Here's how the part is built. I have some questions about the finished solid (model axes, mm). A direction names the side the tool comes from. Coordinates: 2 decimals unless noted, no trailing zeros. Write each loop counter-clockwise with the first axis right and the second up, starting at its lowest first coordinate (ties: lowest second). Pieces come first, ordered by that corner, then holes. Notation, with made-up numbers: (19.25, -10) - (29.25, -10) arc R25 ccw to (29.25, 29) - close; hole circle Ø4 at (58.5, 62). An arc over 180 degrees is marked (long way). Answer in a Markdown table with one row per item. Add a question column.
Item 1: We'd pull the mould along Y, two halves only. Please class faces 1 (the face through (38, 9.7, 1)), 2 (the face through (36, 5.2, 1)), 3 (the face through (34.5, -11, 1)), 4 (the face through (44, -13.7, 1)): +Y half, -Y half, draft (parallel to the pull), parting line (faces both ways), or undercut.
Item 2: Imagine slicing it at D-D (x = 36). Please give me the cut outline in (y, z), plus the area to 3 significant figures.
Item 3: Which directions (+Z, -Z, +X, -X, +Y, -Y) give clear straight access to the entire face, cutting with the end or side of a thin tool? Please do faces 5 (the face through (47, 11.7, 1)), 6 (the face through (37.5, -11, 1)), 7 (the face through (34, -9.7, 1)), 8 (the face through (34.5, 11, 1)).
Item 4: Imagine slicing it at C-C (y = -10.75). Please give me the cut outline in (x, z).
Item 5: Imagine slicing it at B-B (x = 3.5). Please give me the cut outline in (y, z).
Item 6: I'm going to push flat-ended pins straight in: pin 1 (0.6 mm diameter, centred on x = 38.5, z = 0.5, fed in from +Y); pin 2 (7.5 mm diameter, centred on x = 0, y = 0, fed in from -Z); pin 3 (1 mm diameter, centred on y = 12.5, z = 1.5, fed in from +X); pin 4 (0.6 mm diameter, centred on x = 32, z = 1, fed in from -Y). Where does each tip first touch, or does it pass through?
Item 7: Imagine slicing it at A-A (y = 0). Please give me the cut outline in (x, z).
Item 8: If I drill on probe 1 along Y at (x, z) = (0, 0.6); probe 2 along Y at (x, z) = (-3.5, 0.5); probe 3 along X at (y, z) = (-6.5, 0.7), over which ranges is the centre line in solid material (lowest first)? Write a range as from..to.
from build123d import *

# Parameters (mm, degrees)
SKETCH1_R           = 4.05
SKETCH1_R_2         = 1
BOSS_EXTRUDE1_DEPTH = 2


with BuildPart() as part:
    # Sketch1 → Boss-Extrude1 (new body)
    with BuildSketch(Plane.XY):
        with BuildLine():
            Line((48, 11.7), (48, -11.7))
            Line((48, -11.7), (46, -11.7))
            Line((46, -11.7), (46, -13.7))
            Line((46, -13.7), (41, -13.7))
            Line((41, -13.7), (41, -11.7))
            Line((41, -11.7), (37.5, -11.7))
            Line((37.5, -11.7), (37.5, -9.7))
            Line((37.5, -9.7), (38.6, -9.7))
            Line((38.6, -9.7), (38.6, -7.4))
            Line((38.6, -7.4), (37.5, -7.4))
            Line((37.5, -7.4), (37.5, -5.2))
            Line((37.5, -5.2), (34.5, -5.2))
            Line((34.5, -5.2), (34.5, -7.4))
            Line((34.5, -7.4), (33.4, -7.4))
            Line((33.4, -7.4), (33.4, -9.7))
            Line((33.4, -9.7), (34.5, -9.7))
            Line((34.5, -9.7), (34.5, -11.7))
            Line((34.5, -11.7), (31, -11.7))
            Line((31, -11.7), (31, -13.7))
            Line((31, -13.7), (26, -13.7))
            Line((26, -13.7), (26, -11.7))
            Line((26, -11.7), (0, -11.7))
            ThreePointArc((0, -11.7), (-11.7, 0), (0, 11.7))
            Line((0, 11.7), (26, 11.7))
            Line((26, 11.7), (26, 13.7))
            Line((26, 13.7), (31, 13.7))
            Line((31, 13.7), (31, 11.7))
            Line((31, 11.7), (34.5, 11.7))
            Line((34.5, 11.7), (34.5, 9.7))
            Line((34.5, 9.7), (33.4, 9.7))
            Line((33.4, 9.7), (33.4, 7.4))
            Line((33.4, 7.4), (34.5, 7.4))
            Line((34.5, 7.4), (34.5, 5.2))
            Line((34.5, 5.2), (37.5, 5.2))
            Line((37.5, 5.2), (37.5, 7.4))
            Line((37.5, 7.4), (38.6, 7.4))
            Line((38.6, 7.4), (38.6, 9.7))
            Line((38.6, 9.7), (37.5, 9.7))
            Line((37.5, 9.7), (37.5, 11.7))
            Line((37.5, 11.7), (41, 11.7))
            Line((41, 11.7), (41, 13.7))
            Line((41, 13.7), (46, 13.7))
            Line((46, 13.7), (46, 11.7))
            Line((46, 11.7), (48, 11.7))
        make_face()
        Circle(SKETCH1_R, mode=Mode.SUBTRACT)
        with Locations((7, 0)):
            Circle(SKETCH1_R_2, mode=Mode.SUBTRACT)
        with Locations((6.062177826, -3.5)):
            Circle(SKETCH1_R_2, mode=Mode.SUBTRACT)
        with Locations((3.5, -6.062177826)):
            Circle(SKETCH1_R_2, mode=Mode.SUBTRACT)
        with Locations((0, -7)):
            Circle(SKETCH1_R_2, mode=Mode.SUBTRACT)
        with Locations((-3.5, -6.062177826)):
            Circle(SKETCH1_R_2, mode=Mode.SUBTRACT)
        with Locations((-6.062177826, -3.5)):
            Circle(SKETCH1_R_2, mode=Mode.SUBTRACT)
        with Locations((-7, 0)):
            Circle(SKETCH1_R_2, mode=Mode.SUBTRACT)
        with Locations((-6.062177826, 3.5)):
            Circle(SKETCH1_R_2, mode=Mode.SUBTRACT)
        with Locations((-3.5, 6.062177826)):
            Circle(SKETCH1_R_2, mode=Mode.SUBTRACT)
        with Locations((0, 7)):
            Circle(SKETCH1_R_2, mode=Mode.SUBTRACT)
        with Locations((3.5, 6.062177826)):
            Circle(SKETCH1_R_2, mode=Mode.SUBTRACT)
        with Locations((6.062177826, 3.5)):
            Circle(SKETCH1_R_2, mode=Mode.SUBTRACT)
    extrude(amount=BOSS_EXTRUDE1_DEPTH)


solid = part.part
Here are the results:
| question | item | result |
|---|---|---|
| 1 | face 1 | undercut |
| 1 | face 2 | +Y half |
| 1 | face 3 | draft |
| 1 | face 4 | -Y half |
| 2 | outline | (-5.2, 0) - (5.2, 0) - (5.2, 2) - (-5.2, 2) - close |
| 2 | area | 20.8 mm2 |
| 3 | face 5 | +Z, -Z, +X, +Y |
| 3 | face 6 | +Z, -Z, -Y |
| 3 | face 7 | +Z, -Z |
| 3 | face 8 | +Z, -Z, +Y |
| 4 | outline | (-4.62, 0) - (34.5, 0) - (34.5, 2) - (-4.62, 2) - close; (37.5, 0) - (48, 0) - (48, 2) - (37.5, 2) - close |
| 5 | outline | (-11.7, 0) - (-7.06, 0) - (-7.06, 2) - (-11.7, 2) - close; (-5.06, 0) - (-2.04, 0) - (-2.04, 2) - (-5.06, 2) - close; (2.04, 0) - (5.06, 0) - (5.06, 2) - (2.04, 2) - close; (7.06, 0) - (11.7, 0) - (11.7, 2) - (7.06, 2) - close |
| 6 | pin 1 | stops at y = 11.7 |
| 6 | pin 2 | passes through |
| 6 | pin 3 | stops at x = 46 |
| 6 | pin 4 | stops at y = -11.7 |
| 7 | outline | (-11.7, 0) - (-8, 0) - (-8, 2) - (-11.7, 2) - close; (-6, 0) - (-4.05, 0) - (-4.05, 2) - (-6, 2) - close; (4.05, 0) - (6, 0) - (6, 2) - (4.05, 2) - close; (8, 0) - (48, 0) - (48, 2) - (8, 2) - close |
| 8 | probe 1 | y = -11.7..-8, -6..-4.05, 4.05..6, 8..11.7 |
| 8 | probe 2 | y = -11.16..-7.06, -5.06..-2.04, 2.04..5.06, 7.06..11.16 |
| 8 | probe 3 | x = -9.73..-4.4, -2.6..-0.87, 0.87..2.6, 4.4..34.5, 37.5..48 |
